Could you check a few things on this model? Use its own coordinates, in mm. Face numbers are marked on the shaded views. A direction names the side the tool comes from. Coordinates: 2 decimals unless noted, no trailing zeros. Loops run counter-clockwise (first coordinate to the right, second up) from the corner with the lowest first, then second, coordinate; pieces in that order, holes last. Notation, with made-up numbers: (52.25, 78) - (57.25, 78) arc R21 ccw to (57.25, 113) - close; hole circle Ø5 at (57.25, 7.5). An arc over 180 degrees is marked (long way). One line per item, written item: value. Start each with the question number.
(1) If we section it at A-A on z = 0: Write out the boundary of the cut face in (x, y).
(2) If we section it at B-B on y = -1.5: Write out the boundary of the cut face in (x, z).
(3) If we section it at C-C on x = 7.5: Write out the boundary of the cut face in (y, z), then the cut area to 3 significant figures.
(4) If we mould it in two halves opening along X, with no side actions, what happens to the marked faces 1, 2, 3 and 4? For each: pulls with the +X half, pulls with the -X half, needs draft (parallel to the pull), parting line crosses it, or undercut.
(5) I'm going to push flat-ended pins straight in: P1, Ø1.5, axis at x = -8, z = -16, coming from the +Y side; P2, Ø6.5, axis at y = 29.5, z = -6, coming from the -X side; P3, Ø10, axis at x = -15.5, z = -13, coming from the -Y side; P4, Ø3.5, axis at x = -3, y = 48.5, coming from the +Z side. Where does each tip first touch, or does it pass through?
(6) If we section it at D-D on y = 44: Write out the boundary of the cut face in (x, z), then the cut area to 3 significant figures.
(7) On a 3-axis mill with a long thin cutter (end or side, diameter ignored), from which of +Z, -Z, +X, -X, +Y, -Y can I reach the whole of each face in a straight line? I mean the marked faces 5, 6, 7 and 8. Say none if no direction works.
(8) If I drill on line 1 along Z through (x, y) = (-9.5, -2); line 2 along X through (y, z) = (29.5, -2.5); line 3 along X through (y, z) = (-1.65, 0), over which ranges is the centre line in solid material (lowest first)? Write a range as from..to.
Autodesk Fusion 360 part; units mm, degrees
sketch "Sketch1" plane through (0, 0, 0) normal (0, 1, 0) x (1, 0, 0)
  line L0 (20, -20) -> (-20, -20)
  line L1 (-20, -20) -> (-20, 20)
  line L2 (-20, 20) -> (20, 20)
  line L3 (20, 20) -> (20, -20)
  line L4 (20, -20) -> (-20, 20) construction
  line L5 (-20, -20) -> (20, 20) construction
  line L6 (-20, 4) -> (-15, 4)
  line L7 (-15, 4) -> (-15, -4)
  line L8 (-15, -4) -> (-20, -4)
  line L9 (-20, -4) -> (-20, 4)
  line L10 (-4, 20) -> (4, 20)
  line L11 (4, 20) -> (4, 15)
  line L12 (4, 15) -> (-4, 15)
  line L13 (-4, 15) -> (-4, 20)
  line L14 (20, 4) -> (15, 4)
  line L15 (15, 4) -> (15, -4)
  line L16 (15, -4) -> (20, -4)
  line L17 (20, -4) -> (20, 4)
  line L18 (-4, -20) -> (4, -20)
  line L19 (4, -20) -> (4, -15)
  line L20 (4, -15) -> (-4, -15)
  line L21 (-4, -15) -> (-4, -20)
  dimension "d1" = 40
  dimension "d2" = 40
  dimension "d3" = 5
  dimension "d4" = 8
  dimension "d5" = 16
  dimension "d6" = 5
  dimension "d7" = 16
  dimension "d8" = 8
  dimension "d9" = 5
  dimension "d10" = 5
  dimension "d11" = 8
  dimension "d12" = 8
  dimension "d13" = 16
  dimension "d14" = 16
extrude "Extrude1" add sketch "Sketch1" against normal blind 3 contours L0 L1 L2 L3 L6 L7 L8 L11 L12 L13 L14 L15 L16 L19 L20 L21
extrude "Extrude2" add sketch "Sketch1" against normal blind 8 contours L0 L18 L19 L20 L21 | L3 L14 L15 L16 L17 | L1 L6 L7 L8 L9 | L2 L10 L11 L12 L13
hole "Hole1" at (0, 0, 0) direction (0, -1, 0) diameter 9 depth 30 tip angle 118
fillet "Fillet1" radius 4 4 edges at (20, -1.5, -20) (-20, -1.5, -20) (20, -1.5, 20) (-20, -1.5, 20)
sketch "Sketch2" plane through (0, 0, 0) normal (0, 1, 0) x (1, 0, 0)
  line L0 (-10.5, 20) -> (10.5, 20)
  line L1 (10.5, 20) -> (10.5, -1)
  line L2 (10.5, -1) -> (-10.5, -1)
  line L3 (-10.5, -1) -> (-10.5, 20)
  point P0 (-20, 20)
  dimension "d24" = 21
  dimension "d25" = 21
  dimension "d26" = 9.5
extrude "Extrude3" add sketch "Sketch2" along normal blind 50
hole "Hole2" at (0, 0, 0) direction (0, 1, 0) diameter 9 depth 55 tip angle 118 counterbore diameter 13 counterbore depth 27
sketch "Sketch3" plane through (0, -3, 0) normal (0, -1, 0) x (1, 0, 0)
  arc A0 (-16, 20) -> (-20, 16) centre (-16, 16) ccw
  line L0 (-20, 16) -> (-20, 4)
  line L1 (-20, 4) -> (-15, 4)
  line L2 (-15, 4) -> (-15, -4)
  line L3 (-15, -4) -> (-20, -4)
  line L4 (-20, -4) -> (-20, -16)
  arc A1 (-20, -16) -> (-16, -20) centre (-16, -16) ccw
  line L5 (-16, -20) -> (-4, -20)
  line L6 (-4, -20) -> (-4, -15)
  line L7 (-4, -15) -> (4, -15)
  line L8 (4, -15) -> (4, -20)
  line L9 (4, -20) -> (16, -20)
  arc A2 (16, -20) -> (20, -16) centre (16, -16) ccw
  line L10 (20, -16) -> (20, -4)
  line L11 (20, -4) -> (15, -4)
  line L12 (15, -4) -> (15, 4)
  line L13 (15, 4) -> (20, 4)
  line L14 (20, 4) -> (20, 16)
  arc A3 (20, 16) -> (16, 20) centre (16, 16) ccw
  line L15 (16, 20) -> (4, 20)
  line L16 (4, 20) -> (4, 15)
  line L17 (4, 15) -> (-4, 15)
  line L18 (-4, 15) -> (-4, 20)
  line L19 (-4, 20) -> (-16, 20)
  circle A4 centre (0, 0) radius 4.5
  point P0 (-7.5, -4)
  point P1 (7.5, -4)
  dimension "d34" = 16
  dimension "d35" = 15
  dimension "d36" = 12.5
hole "Hole3" at (7.5, -3, -4) at (-7.5, -3, -4) direction (0, 1, 0) diameter 3 depth 55 tip angle 118 counterbore diameter 5 counterbore depth 48
sketch "Sketch4" plane through (0, 50, 0) normal (0, 1, 0) x (-1, 0, 0)
  circle A0 centre (-7.5, -4) radius 1.5
  circle A1 centre (7.5, -4) radius 1.5
  arc A2 (-4.3875, 1) -> (4.3875, 1) centre (0, 0) ccw
  line L0 (-4.3875, 1) -> (-10.5, 1)
  line L1 (-10.5, 1) -> (-10.5, -20)
  line L2 (-10.5, -20) -> (10.5, -20)
  line L3 (10.5, -20) -> (10.5, 1)
  line L4 (10.5, 1) -> (4.3875, 1)
  line L5 (10.5, -20) -> (-10.5, -20)
  line L6 (-10.5, -20) -> (-10.5, 1)
  line L7 (-10.5, 1) -> (10.5, 1)
  line L8 (10.5, 1) -> (10.5, -20)
  line L9 (-8.5, -18) -> (-8.5, -1)
  line L10 (-8.5, -1) -> (8.5, -1)
  line L11 (8.5, -1) -> (8.5, -18)
  line L12 (8.5, -18) -> (-8.5, -18)
  line L13 (8.5, -18) -> (-8.5, -18)
  line L14 (-8.5, -18) -> (-8.5, -6.8913)
  line L15 (-8.5, -6.8913) -> (8.5, -6.8913)
  line L16 (8.5, -6.8913) -> (8.5, -18)
  dimension "d42" = 2
extrude "Extrude4" cut sketch "Sketch4" against normal blind 3 contours L9 L11 L12 L13 L14 L15 L16
equation "d6 = d3"
equation "d7 = d5"
equation "d8 = d4"
equation "d9 = d3"
equation "d10 = d3"
equation "d11 = d4"
equation "d12 = d4"
equation "d13 = d7"
equation "d14 = d7"
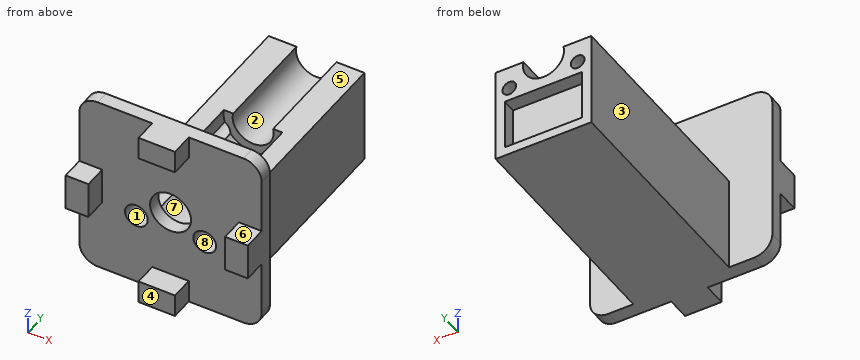
Values:
1. outline: (-20, -8) - (-15, -8) - (-15, -3) - (-4.5, -3) - (-4.5, 0) - (-6.5, 0) - (-6.5, 27) - (-4.5, 27) - (-4.5, 50) - (-10.5, 50) - (-10.5, 0) - (-20, 0) - close; (4.5, -3) - (15, -3) - (15, -8) - (20, -8) - (20, 0) - (10.5, 0) - (10.5, 50) - (4.5, 50) - (4.5, 27) - (6.5, 27) - (6.5, 0) - (4.5, 0) - close
2. outline: (-20, -16) arc R4 ccw to (-16, -20) - (16, -20) arc R4 ccw to (20, -16) - (20, 16) arc R4 ccw to (16, 20) - (-16, 20) arc R4 ccw to (-20, 16) - close; hole circle Ø5 at (-7.5, -4); hole circle Ø9 at (0, 0); hole circle Ø5 at (7.5, -4)
3. outline: (-3, -20) - (50, -20) - (50, -18) - (47, -18) - (47, -6.89) - (50, -6.89) - (50, -5.5) - (45, -5.5) - (45, -6.5) - (-3, -6.5) - close; (-3, -1.5) - (45, -1.5) - (45, -2.5) - (50, -2.5) - (50, 1) - (0, 1) - (0, 20) - (-3, 20) - close
3. area: 882 mm2
4. face 1: undercut
4. face 2: undercut
4. face 3: pulls with the -X half
4. face 4: needs draft
5. P1: stops at y = 50
5. P2: stops at x = -10.5
5. P3: stops at y = -3
5. P4: stops at z = 1
6. outline: (-10.5, -20) - (10.5, -20) - (10.5, 1) - (4.39, 1) arc R4.5 cw (long way) to (-4.39, 1) - (-10.5, 1) - close; hole circle Ø5 at (-7.5, -4); hole circle Ø5 at (7.5, -4)
6. area: 361 mm2
7. face 5: +Z, +X, -X, +Y
7. face 6: +Z, +X, -X, -Y
7. face 7: +Z
7. face 8: -Y
8. line 1: z = -20..-5.5, -2.5..20
8. line 2: x = -10.5..-9.5, -5.5..-3.74, 3.74..5.5, 9.5..10.5
8. line 3: x = -20..-4.5, 4.5..20
